Read the model definition and answer for the solid it produces. Units are mm, in the model's axes. A direction names the side the tool comes from. Coordinates: 2 decimals unless noted, no trailing zeros. Loops run counter-clockwise (first coordinate to the right, second up) from the corner with the lowest first, then second, coordinate; pieces in that order, holes last. Notation, with made-up numbers: M 80.25,-27.75 L 114.25,-27.75 A15 ccw 114.25,-23.75 Z; hole C 54,57 d6. An arc over 180 degrees is marked long. Put each result on its own line as item: value.
from build123d import *

# Parameters (mm, degrees)
PAD_DEPTH = 2


with BuildPart() as part:
    # Sketch (on Face1 of CopyPad007) → Pad (new body)
    with BuildSketch(Plane.XY.offset(82)):
        Polygon((15, 4), (15, 12), (21, 12), (21, 51), (99, 51), (99, 12), (105, 12), (105, 4), align=None)
    extrude(amount=PAD_DEPTH)


with BuildPart() as part_1:
    # Body001 placement: moved
    add(part.part.moved(Location((7.386589, 4.959148, 2.147461))))


solid = part_1.part
1) Find section A-A, the plane z = 85.7. Write down the section's boundary in (x, y), plus the area to 3 significant figures.
Answer list:
outline: M 22.39,8.96 L 112.39,8.96 L 112.39,16.96 L 106.39,16.96 L 106.39,55.96 L 28.39,55.96 L 28.39,16.96 L 22.39,16.96 Z
area: 3,760 mm^2
2) Find section C-C, the plane x = 107.5. Write down the section's boundary in (y, z), plus the area to 3 significant figures.
Answer list:
outline: M 8.96,84.15 L 16.96,84.15 L 16.96,86.15 L 8.96,86.15 Z
area: 16.0 mm^2
3) A straight line is drawn through the part: line 1 (X direction, y = 28.5, z = 85.1). Find the intervals that lie inside material, in ascending order. Write a range as [from, to].
Answer list:
line 1: x = [28.39, 106.39]
4) Given pin 1 Ø1 at (y, z) = (37.5, 85.5) entering from -X; pin 2 Ø1 at (x, z) = (25.5, 85) entering from +Y, each flat-ended and moving along its own axis, determine where each tip first touches the part or whether it passes through.
Answer list:
pin 1: stops at x = 28.39
pin 2: stops at y = 16.96
5) Find section B-B, the plane y = 52. Write down the section's boundary in (x, z), plus the area to 3 significant figures.
Answer list:
outline: M 28.39,84.15 L 106.39,84.15 L 106.39,86.15 L 28.39,86.15 Z
area: 156 mm^2
6) Which of the six approach directions +Z, -Z, +X, -X, +Y, -Y give full straight-line access (tool end or side, diameter ignored) to faces 1 (the flat face through (28.387, 36, 85)), 2 (the flat face through (67, 55.959, 85)), 3 (the flat face through (106.387, 37, 85))?
Answer list:
face 1: +Z, -Z, -X, +Y
face 2: +Z, -Z, +X, -X, +Y
face 3: +Z, -Z, +X, +Y
